from build123d import *

# Parameters (mm, degrees)
SKETCH1_R                 = 9
SEAL_CONE_DEPTH           = 24.278516115
SEAL_CONE_DRAFT           = -35
SKETCH2_R                 = 7
CONE_HOLLOW_DEPTH         = 24.278516115
CONE_HOLLOW_DRAFT         = -35
SKETCH3_R                 = 29
TOP_PLATE_DEPTH           = 3
SKETCH4_W                 = 33.5
SKETCH4_H                 = 23.5
MQ3_PCB_POCKET_DEPTH      = 1.25
SKETCH5_R                 = 10.3
SKETCH5_R_2               = 4.1
SKETCH5_R_3               = 1
CAN_HOSE_VENT_HOLES_DEPTH = 1.9


with BuildPart() as part:
    # Sketch1 → Seal_cone (with draft: the straight prism first)
    with BuildSketch(Plane.XY):
        Circle(SKETCH1_R)
    extrude(amount=SEAL_CONE_DEPTH)
    # Seal_cone: the draft: its side faces are tilted about the plane it starts from
    seal_cone_sides = [part.faces().sort_by_distance(p)[0] for p in [
        (-9, 0, 12.139258057),
    ]]
    draft(seal_cone_sides, Plane.XY, SEAL_CONE_DRAFT)


with BuildPart() as cone_hollow_tool:
    # Sketch2 → Cone_hollow (with draft: the straight prism first)
    with BuildSketch(Plane.XY):
        Circle(SKETCH2_R)
    extrude(amount=CONE_HOLLOW_DEPTH)
    # Cone_hollow: the draft: its side faces are tilted about the plane it starts from
    cone_hollow_sides = [cone_hollow_tool.faces().sort_by_distance(p)[0] for p in [
        (-7, 0, 12.139258057),
    ]]
    draft(cone_hollow_sides, Plane.XY, CONE_HOLLOW_DRAFT)


with BuildPart() as part_1:
    add(part.part)

    # Cone_hollow: cut by cone_hollow_tool
    add(cone_hollow_tool.part, mode=Mode.SUBTRACT)

    # Sketch3 → Top_plate (add)
    with BuildSketch(Plane.XY.offset(24.278516115)):
        Circle(SKETCH3_R)
    extrude(amount=TOP_PLATE_DEPTH)

    # Sketch4 → MQ3_pcb_pocket (cut, symmetric)
    with BuildSketch(Plane.XY.offset(26.528516115)):
        Rectangle(SKETCH4_W, SKETCH4_H)
    extrude(amount=MQ3_PCB_POCKET_DEPTH, both=True, mode=Mode.SUBTRACT)

    # Sketch5 → Can_hose_vent_holes (cut, symmetric)
    with BuildSketch(Plane.XY.offset(25.878516115)):
        Circle(SKETCH5_R)
        with Locations((0, 18)):
            Circle(SKETCH5_R_2)
        with Locations((0, -18)):
            Circle(SKETCH5_R_3)
    extrude(amount=CAN_HOSE_VENT_HOLES_DEPTH, both=True, mode=Mode.SUBTRACT)


solid = part_1.part
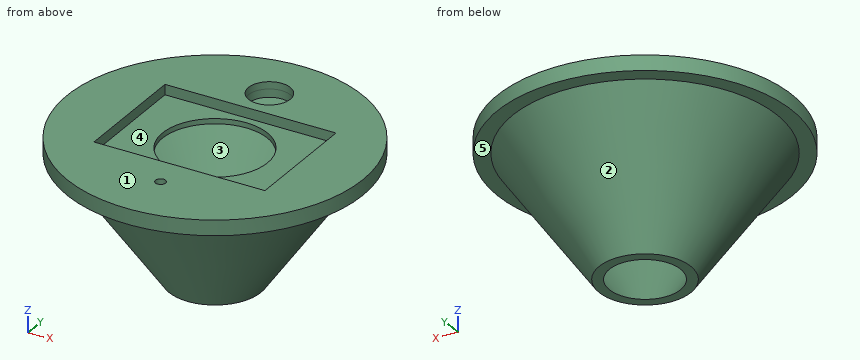
CAD build for the part. Positions are in the model's coordinates, mm. Face numbers are marked on the shaded views. A direction names the side the tool comes from. Coordinates: 2 decimals unless noted, no trailing zeros. Write each loop counter-clockwise with the first axis right and the second up, starting at its lowest first coordinate (ties: lowest second). Pieces come first, ordered by that corner, then holes. Notation, with made-up numbers: (-8.5, 14.5) - (30.5, 14.5) arc R21 ccw to (30.5, 49.5) - close; hole circle Ø9 at (55, -25). An arc over 180 degrees is marked (long way). Use a Markdown table: item, result. Add a question column.
Item 1: 3-axis set-ups, long thin cutter, end or side, ignore diameter. For the marked faces 4 and 5: which of +Z, -Z, +X, -X, +Y, -Y reach the whole face in a straight line?
Item 2: Band-saw the part on C-C, the plane z = 12. Give the cut face in (x, y), and give its area (3 significant figures).
Item 3: Mould opens along Z. For the marked faces 1, 2 and 3 say: pulls with the +Z half, pulls with the -Z half, needs draft (parallel to the pull), parting line crosses it, or undercut.
Item 4: Band-saw the part on D-D, the plane z = 2. Give the cut face in (x, y), and give its area (3 significant figures).
Item 5: Band-saw the part on A-A, the plane x = 0. Give the cut face in (y, z), and give its area (3 significant figures).
Item 6: Band-saw the part on B-B, the plane y = 0. Give the cut face in (x, z), and give its area (3 significant figures).
Item 7: Drill centre lines: L1, parallel to Y at x = 0, z = 26.95; L2, parallel to Y at x = 0, z = 25; L3, parallel to Z at x = 17.5, y = -21. Where is each one in solid material? Low to high. Write a range as from..to.
Item 8: Flat gauge pins, fed straight in: pin 1 (0.6 mm diameter, centred on x = -6.5, z = 26, fed in from -Y); pin 2 (1.5 mm diameter, centred on x = -3.5, y = -12, fed in from -Z); pin 3 (6.5 mm diameter, centred on x = 0, y = 18, fed in from +Z). Where does each tip first touch, or does it go through?
Numbers:
| question | item | result |
|---|---|---|
| 1 | face 4 | +Z |
| 1 | face 5 | -Z |
| 2 | outline | circle Ø34.8 at (0, 0); hole circle Ø30.8 at (0, 0) |
| 2 | area | 206 mm2 |
| 3 | face 1 | pulls with the +Z half |
| 3 | face 2 | pulls with the -Z half |
| 3 | face 3 | undercut |
| 4 | outline | circle Ø20.8 at (0, 0); hole circle Ø16.8 at (0, 0) |
| 4 | area | 118 mm2 |
| 5 | outline | (-29, 24.28) - (-26, 24.28) - (-9, 0) - (-7, 0) - (-24, 24.28) - (-19, 24.28) - (-19, 27.28) - (-29, 27.28) - close; (-17, 24.28) - (-10.3, 24.28) - (-10.3, 25.28) - (-11.75, 25.28) - (-11.75, 27.28) - (-17, 27.28) - close; (7, 0) - (9, 0) - (26, 24.28) - (29, 24.28) - (29, 27.28) - (22.1, 27.28) - (22.1, 24.28) - (24, 24.28) - close; (10.3, 24.28) - (13.9, 24.28) - (13.9, 27.28) - (11.75, 27.28) - (11.75, 25.28) - (10.3, 25.28) - close |
| 5 | area | 173 mm2 |
| 6 | outline | (-29, 24.28) - (-26, 24.28) - (-9, 0) - (-7, 0) - (-24, 24.28) - (-10.3, 24.28) - (-10.3, 25.28) - (-16.75, 25.28) - (-16.75, 27.28) - (-29, 27.28) - close; (7, 0) - (9, 0) - (26, 24.28) - (29, 24.28) - (29, 27.28) - (16.75, 27.28) - (16.75, 25.28) - (10.3, 25.28) - (10.3, 24.28) - (24, 24.28) - close |
| 6 | area | 184 mm2 |
| 7 | L1 | -29..-19, -17..-11.75, 11.75..13.9, 22.1..29 |
| 7 | L2 | -29..-19, -17..-10.3, 10.3..13.9, 22.1..29 |
| 7 | L3 | 24.28..27.28 |
| 8 | pin 1 | y = -28.33 |
| 8 | pin 2 | z = 3.93 |
| 8 | pin 3 | z = 20.35 |
